from build123d import *

# Parameters (mm, degrees)
F2_R     = 3.55
F3_DEPTH = 20.5
F5_DEPTH = 9
F6_R     = 0.5
F7_R     = 1.2
F8_DEPTH = 25


with BuildPart() as f1:
    # F0 (on Front) → F1 (revolve)
    with BuildSketch(Plane.XZ):
        Polygon((-6, 0), (0, 0), (0, 21.5), (-9, 21.5), (-9, 6.5), (-5, 6.5), (-5, 2), (-6, 2), align=None)
    revolve(axis=Axis((0, 0, -3.667768), (0, 0, -1)))

    # F2 (on face) → F3 (cut)
    with BuildSketch(Plane(origin=(0, 0, 0), x_dir=(1, 0, 0), z_dir=(0, 0, -1))):
        Circle(F2_R)
    extrude(amount=-F3_DEPTH, mode=Mode.SUBTRACT)

    # F4 (on face) → F5 (join)
    with BuildSketch(Plane(origin=(0, 0, 20.5), x_dir=(1, 0, 0), z_dir=(0, 0, -1))):
        with BuildLine():
            Line((3.207453, -1.521429), (-3.207453, -1.521429))
            ThreePointArc((-3.207453, -1.521429), (0, -3.55), (3.207453, -1.521429))
        make_face()
    extrude(amount=F5_DEPTH)

    # F6
    f6_edges = [f1.edges().sort_by_distance(p)[0] for p in [
        (9, 0, 21.5),
    ]]
    fillet(f6_edges, radius=F6_R)

    # F7 (on face) → F8 (cut)
    with BuildSketch(Plane.XZ.offset(-1.521429)):
        with Locations((0, 14.5)):
            Circle(F7_R)
    extrude(amount=-F8_DEPTH, mode=Mode.SUBTRACT)


solid = f1.part
Could you check a few things on this model? Use its own coordinates, in mm. A direction names the side the tool comes from. Round coordinates to 2 decimals unless told otherwise and drop trailing zeros. Order: outer loops, then holes, each group sorted by start corner. A loop starts at its lowest first (then second) coordinate and runs counter-clockwise, first axis right, second up.
Q1. Which directions (+Z, -Z, +X, -X, +Y, -Y) give clear straight access to the entire face, cutting with the end or side of a thin tool? Please do faces 1 (the face through (-3, -3, 0)), 2 (the face through (-4, -4, 6.5)), 3 (the face through (-0.26, 5.21, 13.33)), 4 (the face through (1.172, 8.923, 13.648)), 5 (the face through (-0.46, -3.52, 10.11)).
Geometry says:
face 1: -Z, +X, -X, +Y, -Y
face 2: none
face 3: +Y
face 4: +Z, -Z
face 5: -Z
Q2. Imagine slicing it at D-D, the plane z = 1.5. List the corners of the cut face in (x, y) for me, then the cut area to 3 significant figures.
Geometry says:
outline: circle Ø12 at (0, 0); hole circle Ø7.1 at (0, 0)
area: 73.5 mm2
Q3. Please list where these lines run through material, in increasing order: probe 1 along Z at (x, y) = (-3.5, 4.75); probe 2 along Z at (x, y) = (0, 3.75); probe 3 along Y at (x, z) = (0, 10.5).
Geometry says:
probe 1: z = 0 to 2, 6.5 to 21.5
probe 2: z = 0 to 13.3, 15.7 to 21.5
probe 3: y = -9 to -3.55, 3.55 to 9
Q4. Thinking about a two-plate mould opening in X: for faces 6 (the face through (1.08, -4.88, 4.22)), 7 (the face through (0, 0, 21.5)), 8 (the face through (0, 0, 20.5)), which applies, released by +X, released by -X, zero draft, split by the parting line, or undercut?
Geometry says:
face 6: split by the parting line
face 7: zero draft
face 8: undercut
Q5. Imagine slicing it at C-C, the plane z = 14.5. List the corners of the cut face in (x, y) for me, then the cut area to 3 significant figures.
Geometry says:
outline: (-3.21, 1.52) - (-1.2, 1.52) - (-1.2, 8.92) arc R9 ccw (long way) to (1.2, 8.92) - (1.2, 1.52) - (3.21, 1.52) arc R3.55 cw (long way) to start
area: 206 mm2
Q6. I'm going to push flat-ended pins straight in: P1, Ø1.5, axis at x = -1.5, y = 0, coming from the -Z side; P2, Ø1, axis at x = 5, y = 5.5, coming from the -Z side; P3, Ø5.5, axis at x = 0, y = 0, coming from the -Z side. Where does each tip first touch, or does it pass through?
Geometry says:
P1: stops at z = 20.5
P2: stops at z = 6.5
P3: stops at z = 11.5
Q7. Imagine slicing it at B-B, the plane z = 12.25. List the corners of the cut face in (x, y) for me, then the cut area to 3 significant figures.
Geometry says:
outline: circle Ø18 at (0, 0); hole (-3.21, 1.52) arc R3.55 ccw (long way) to (3.21, 1.52) - close
area: 224 mm2
Q8. Imagine slicing it at A-A, the plane x = 0. List the corners of the cut face in (y, z) for me.
Geometry says:
outline: (-9, 6.5) - (-5, 6.5) - (-5, 2) - (-6, 2) - (-6, 0) - (-3.55, 0) - (-3.55, 20.5) - (1.52, 20.5) - (1.52, 15.7) - (9, 15.7) - (9, 21) arc R0.5 ccw to (8.5, 21.5) - (-8.5, 21.5) arc R0.5 ccw to (-9, 21) - close; (1.52, 11.5) - (3.55, 11.5) - (3.55, 0) - (6, 0) - (6, 2) - (5, 2) - (5, 6.5) - (9, 6.5) - (9, 13.3) - (1.52, 13.3) - close
